```python
from build123d import *

# Parameters (mm, degrees)
F0_R      = 20
F1_DEPTH  = 7.6
F3_DEPTH  = 3.9
F4_W      = 7.6
F4_H      = 3
F5_W      = 7.6
F5_H      = 3
F6_DEPTH  = 4.4
F7_W      = 7.6
F7_H      = 7.8
F8_DEPTH  = 0.5
F11_DEPTH = 3.55
F12_R     = 2.725
F13_DEPTH = 7.6


with BuildPart() as f1:
    # F0 (on Top) → F1 (new body)
    with BuildSketch(Plane.XY):
        Circle(F0_R)
    extrude(amount=-F1_DEPTH)

    # F2 (on face) → F3 (cut)
    with BuildSketch(Plane.XY):
        with BuildLine():
            Line((19.6160648449, 3.9), (-19.6160648449, 3.9))
            ThreePointArc((-19.6160648449, 3.9), (-20, 0), (-19.6160648449, -3.9))
            Line((-19.6160648449, -3.9), (19.6160648449, -3.9))
            ThreePointArc((19.6160648449, -3.9), (19.903784777, -1.9594263321), (20, 0))
            ThreePointArc((20, 0), (19.903784777, 1.9594263321), (19.6160648449, 3.9))
        make_face()
    extrude(amount=-F3_DEPTH, mode=Mode.SUBTRACT)

    # F4 (on face) + F5 (on face) → F6 (cut)
    with BuildSketch(Plane.XY):
        with Locations((0, -5.4)):
            Rectangle(F4_W, F4_H)
    with BuildSketch(Plane.XY):
        with Locations((0, 5.4)):
            Rectangle(F5_W, F5_H)
    extrude(amount=-F6_DEPTH, mode=Mode.SUBTRACT)

    # F7 (on face) → F8 (cut)
    with BuildSketch(Plane.XY.offset(-3.9)):
        Rectangle(F7_W, F7_H)
    extrude(amount=-F8_DEPTH, mode=Mode.SUBTRACT)

    # F10 (on offset) → F11 (join)
    with BuildSketch(Plane.XY.offset(-7.6)):
        Polygon((1.225, 19.8352728039), (1.225, 19.9624491233), (1.225, 25.2124491233), (-6.825, 25.2124491233), (-6.825, 21.2124491233), (-4.375, 21.2124491233), (-4.375, 22.4624491233), (-1.225, 22.4624491233), (-1.225, 19.9624491233), (-1.225, 19.7902154177), align=None)
    extrude(amount=F11_DEPTH)

    # F12 (on face) → F13 (cut)
    with BuildSketch(Plane(origin=(0, 0, -7.6), x_dir=(1, 0, 0), z_dir=(0, 0, -1))):
        Circle(F12_R)
    extrude(amount=-F13_DEPTH, mode=Mode.SUBTRACT)


solid = f1.part
```
Geometry check sheet. Reference: the model listing, model coordinates, mm. A direction names the side the tool comes from. Round coordinates to 2 decimals unless told otherwise and drop trailing zeros. Loops run counter-clockwise (first coordinate to the right, second up) from the corner with the lowest first, then second, coordinate; pieces in that order, holes last. Notation, with made-up numbers: (28, 82.5) - (84, 82.5) arc R12 cw to (84, 103.5) - close; hole circle Ø1 at (9, 56). An arc over 180 degrees is marked (long way). Write each question's results on one line, items separated by ' | '. Start each with the question number.
Q1. Thickness scan on line 1 (Y direction, x = 0, z = -5.1) (3 decimals); line 2 (Y direction, x = -2, z = -5); line 3 (X direction, y = 0, z = -6.1) (3 decimals). Record the ranges inside material, lowest first. Write a range as [from, to].
Q2. Cross-section at C-C on z = -6.5. Enter the section's corners in (x, y) (3 decimals), and give its area (3 significant figures).
Q3. Cross-section at A-A on y = 0. Enter the section's corners in (x, z) (3 decimals).
Q4. Release check for a two-part mould opening along X. For faces 1 (the flat face through (0, 6.9, -2)), 2 (the cylindrical face through (2.6, -0.82, -6.02)), 3 (the flat face through (-6.825, 23, -6)), 4 (the flat face through (-6, 21.212, -6)) record: +X half, -X half, draft (parallel to the pull), parting line (faces both ways), or undercut.
Q5. Cross-section at B-B on x = 0. Enter the section's corners in (y, z) (3 decimals).
Q6. Cross-section at D-D on y = -6. Enter the section's corners in (x, z).
Q7. Gauge pin test, flat ends, axial feed: P1, Ø3, axis at x = -11.5, z = -2, coming from the +Y side; P2, Ø4, axis at x = 8, y = 1, coming from the +Z side; P3, Ø3, axis at x = -8.5, z = -2, coming from the -Y side (3 decimals); P4, Ø3.5, axis at x = 0, y = 0, coming from the -Z side. Record the tip position at first contact, or that the pin passes through.
Q8. Access from +Z, -Z, +X, -X, +Y, -Y to the whole of each face (thin tool, end or side, straight path). Record for faces 5 (the flat face through (-3.8, -0.1, -4.1)), 6 (the flat face through (12, -3.9, -2)), 7 (the flat face through (1.225, 23, -6)), 8 (the flat face through (-3, 22.462, -6)).
Answers below:
1) line 1: y = [-20, -2.725], [2.725, 25.212] | line 2: y = [-19.9, -1.85], [1.85, 19.9], [22.46, 25.21] | line 3: x = [-20, -2.725], [2.725, 20]
2) outline: (-6.825, 21.212) - (-4.375, 21.212) - (-4.375, 22.462) - (-1.225, 22.462) - (-1.225, 19.962) arc R20 ccw (long way) to (1.225, 19.962) - (1.225, 25.212) - (-6.825, 25.212) - close; hole circle Ø5.45 at (0, 0) | area: 1,260 mm²
3) outline: (-20, -7.6) - (-2.725, -7.6) - (-2.725, -4.4) - (-3.8, -4.4) - (-3.8, -3.9) - (-20, -3.9) - close; (2.725, -7.6) - (20, -7.6) - (20, -3.9) - (3.8, -3.9) - (3.8, -4.4) - (2.725, -4.4) - close
4) face 1: undercut | face 2: undercut | face 3: -X half | face 4: draft
5) outline: (-20, -7.6) - (-2.725, -7.6) - (-2.725, -4.4) - (-6.9, -4.4) - (-6.9, 0) - (-20, 0) - close; (2.725, -7.6) - (25.212, -7.6) - (25.212, -4.05) - (20, -4.05) - (20, 0) - (6.9, 0) - (6.9, -4.4) - (2.725, -4.4) - close
6) outline: (-19.08, -7.6) - (19.08, -7.6) - (19.08, 0) - (3.8, 0) - (3.8, -4.4) - (-3.8, -4.4) - (-3.8, 0) - (-19.08, 0) - close
7) P1: stops at y = 17.32 | P2: stops at z = -3.9 | P3: stops at y = -18.735 | P4: passes through
8) face 5: +Z | face 6: +Z, +X, -X | face 7: +Z, -Z, +X, +Y | face 8: +Z, -Z
